Model file for the job. Use its own axes, mm. A direction names the side the tool comes from. Round coordinates to 2 decimals unless told otherwise and drop trailing zeros. Loops run counter-clockwise (first coordinate to the right, second up) from the corner with the lowest first, then second, coordinate; pieces in that order, holes last. Notation, with made-up numbers: M -26,59.5 L 21,59.5 A24 cw 21,96.5 Z; hole C -16,14.5 d1. An arc over 180 degrees is marked long. Use a Markdown table: item, result. Add a question column.
Item 1: Pin check, flat tips, straight feed: P1, Ø4.5, axis at y = 1245, z = 8.5, coming from the +X side; P2, Ø3, axis at y = 1225.5, z = 7.5, coming from the +X side. Stop position of each tip, or through.
Item 2: Saw through at A-A on x = 140. Give the number of separate pieces and of enclosed holes in the cut face, then the cut area to 3 significant figures.
Item 3: Two-plate mould, pull along Y, no slides. Class faces 3 (the flat face through (6, 172, 13.5)), 4 (the flat face through (13, 931, 0)): +Y half, -Y half, draft (parallel to the pull), parting line (faces both ways), or undercut.
Item 4: Saw through at C-C on x = 544.5. Write the cut outline in (y, z).
Item 5: Saw through at B-B on y = 1413. Write the cut outline in (x, z), then the cut area to 3 significant figures.
Item 6: Wall check: L1, parallel to X at y = 1241.5, z = 1.05; L2, parallel to Y at x = 655, z = 0.7; L3, parallel to Z at x = 209, y = 1243.5. Give the ranges that are in metal, low to high. Write a range as from..to.
Item 7: Tool access for faces 1 (the flat face through (13, 939, 15)), 2 (the flat face through (6, 313, 1.5)): list every direction of +Z, -Z, +X, -X, +Y, -Y with a clear straight run to the whole face (end or side of a thin tool).
```python
from build123d import *

# Parameters (mm, degrees)
F1_W      = 15
F1_H      = 15
F1_W_2    = 12
F1_H_2    = 12
F4_W      = 15
F4_H      = 15
F5_DEPTH  = 1.5
F6_W      = 15
F6_H      = 15
F7_DEPTH  = 1.5
F8_R      = 4
F9_DEPTH  = 15
F10_R     = 4
F11_DEPTH = 15


with BuildPart() as f2:
    # F2: sweep along a path in F0
    with BuildLine(Plane.XY) as f2_path:
        Line((310, 0), (0, 0))
        Line((0, 0), (0, 1870))
        Line((0, 1870), (800, 1870))
    # F1 (on Right) → F2 (sweep)
    with BuildSketch(Plane.YZ):
        with Locations((7.5, 7.5)):
            Rectangle(F1_W, F1_H)
        with Locations((7.5, 7.5)):
            Rectangle(F1_W_2, F1_H_2, mode=Mode.SUBTRACT)
    sweep(path=f2_path.line, transition=Transition.RIGHT)

    # F3: sweep along a path in F0
    with BuildLine(Plane.XY) as f3_path:
        Line((0, 628.5), (310, 628.5))
    # F1 (on Right) → F3 (sweep)
    with BuildSketch(Plane.YZ):
        with Locations((628.5, 7.5)):
            Rectangle(F1_W, F1_H)
        with Locations((628.5, 7.5)):
            Rectangle(F1_W_2, F1_H_2, mode=Mode.SUBTRACT)
        with Locations((1241.5, 7.5)):
            Rectangle(F1_W, F1_H)
        with Locations((1241.5, 7.5)):
            Rectangle(F1_W_2, F1_H_2, mode=Mode.SUBTRACT)
    sweep(path=f3_path.line)

    # F4 (on face) → F5 (join)
    with BuildSketch(Plane.YZ.offset(310)):
        with Locations((7.5, 7.5)):
            Rectangle(F4_W, F4_H)
        with Locations((628.5, 7.5)):
            Rectangle(F4_W, F4_H)
        with Locations((1241.5, 7.5)):
            Rectangle(F4_W, F4_H)
    extrude(amount=-F5_DEPTH)

    # F6 (on face) → F7 (join)
    with BuildSketch(Plane.YZ.offset(800)):
        with Locations((1862.5, 7.5)):
            Rectangle(F6_W, F6_H)
    extrude(amount=-F7_DEPTH)

    # F8 (on face) → F9 (cut, through all)
    with BuildSketch(Plane.XY.offset(15)):
        with Locations((290, 628.5)):
            Circle(F8_R)
        with Locations((240, 628.5)):
            Circle(F8_R)
        with Locations((290, 1241.5)):
            Circle(F8_R)
        with Locations((240, 1241.5)):
            Circle(F8_R)
        with Locations((780, 1862.5)):
            Circle(F8_R)
        with Locations((655, 1862.5)):
            Circle(F8_R)
        with Locations((505, 1862.5)):
            Circle(F8_R)
    extrude(amount=-F9_DEPTH, mode=Mode.SUBTRACT)

    # F10 (on face) → F11 (cut, through all)
    with BuildSketch(Plane.XZ):
        with Locations((290, 7.5)):
            Circle(F10_R)
        with Locations((240, 7.5)):
            Circle(F10_R)
        with Locations((45, 7.5)):
            Circle(F10_R)
    extrude(amount=-F11_DEPTH, mode=Mode.SUBTRACT)


solid = f2.part
```
Entries:
| question | item | result |
|---|---|---|
| 1 | P1 | x = 310 |
| 1 | P2 | x = 15 |
| 2 | separate pieces | 4 |
| 2 | enclosed holes | 4 |
| 2 | area | 324 mm2 |
| 3 | face 3 | undercut |
| 3 | face 4 | draft |
| 4 | outline | M 1855,0 L 1870,0 L 1870,15 L 1855,15 Z; hole M 1856.5,1.5 L 1868.5,1.5 L 1868.5,13.5 L 1856.5,13.5 Z |
| 5 | outline | M 0,0 L 15,0 L 15,15 L 0,15 Z; hole M 1.5,1.5 L 13.5,1.5 L 13.5,13.5 L 1.5,13.5 Z |
| 5 | area | 81.0 mm2 |
| 6 | L1 | 0..236, 244..286, 294..310 |
| 6 | L2 | 1855..1858.5, 1866.5..1870 |
| 6 | L3 | 0..1.5, 13.5..15 |
| 7 | face 1 | +Z, +X, -X, +Y, -Y |
| 7 | face 2 | none |
